Autodesk Inventor part; units mm, degrees
ref_plane "YZ Plane" through (0, 0, 0) normal (1, 0, 0) x (0, 1, 0)
ref_plane "XZ Plane" through (0, 0, 0) normal (0, 1, 0) x (-1, 0, 0)
ref_plane "XY Plane" through (0, 0, 0) normal (0, 0, 1) x (1, 0, 0)
sketch "Sketch1" plane through (0, 0, 0) normal (0, 0, 1) x (1, 0, 0)
  line L0 (3.6662, 6.35) -> (7.3323, 0)
  line L1 (7.3323, 0) -> (3.6662, -6.35)
  line L2 (3.6662, -6.35) -> (-3.6662, -6.35)
  line L3 (-3.6662, -6.35) -> (-7.3323, 0)
  line L4 (-7.3323, 0) -> (-3.6662, 6.35)
  line L5 (-3.6662, 6.35) -> (3.6662, 6.35)
  point P0 (0, 0)
  point P1 (0, 0)
  dimension "d0" = 12.7
extrude "Extrusion1" add sketch "Sketch1" along normal blind 228.6
ref_plane "Work Plane1" through (-3.6662, -6.35, 0) normal (-0.866, 0.5, 0) x (0, 0, 1)
ref_plane "Work Plane2" through (-7.3323, 0, 0) normal (0, 1, 0) x (0, 0, 1)
properties part number "Steel Shaft" material "Steel"
Input: part model. Units: mm. Frame: model coordinates. Round coordinates to 2 decimals unless told otherwise and drop trailing zeros. Loops run counter-clockwise (first coordinate to the right, second up) from the corner with the lowest first, then second, coordinate; pieces in that order, holes last. Notation, with made-up numbers: M -33.5,-5.5 L 10.5,-5.5 A27 cw 10.5,12.5 Z; hole C 25.25,58 d11. An arc over 180 degrees is marked long. Answer as CSV lines item,"result". Start each with the question number.
(1) First-contact query: pin 1 (5 mm diameter, centred on y = 3, z = 67.5, fed in from -X); pin 2 (2 mm diameter, centred on y = 3, z = 160, fed in from +X). Flat tips, straight axial feed; report the tip coordinate or a pass-through.
(2) Line query: line 1 (X direction, y = -1.75, z = 59); line 2 (Y direction, x = -4.5, z = 27.5); line 3 (X direction, y = -1.5, z = 203.5). Output: solid intervals per line, ascending. Write a range as [from, to].
(3) Section B-B, the plane y = 4.5. Output: boundary loops of the cut face in (x, z).
(4) Section A-A, the plane z = 117. Output: boundary loops of the cut face in (x, y).
Values found:
1,pin 1,"stops at x = -7.04"
1,pin 2,"stops at x = 6.18"
2,line 1,"x = [-6.32, 6.32]"
2,line 2,"y = [-4.91, 4.91]"
2,line 3,"x = [-6.47, 6.47]"
3,outline,"M -4.73,0 L 4.73,0 L 4.73,228.6 L -4.73,228.6 Z"
4,outline,"M -7.33,0 L -3.67,-6.35 L 3.67,-6.35 L 7.33,0 L 3.67,6.35 L -3.67,6.35 Z"
